```python
from build123d import *

# Parameters (mm, degrees)
F0_R     = 34.9
F0_R_2   = 5.1
F1_DEPTH = 9
F2_R     = 8
F3_DEPTH = 10
F5_DEPTH = 10


# Not quite as in the source:
# - a feature names something its author has since deleted; it is built from what else it names


with BuildPart() as f1:
    # F0 (on Front) → F1 (new body)
    with BuildSketch(Plane.XZ):
        Circle(F0_R)
        Circle(F0_R_2, mode=Mode.SUBTRACT)
    extrude(amount=-F1_DEPTH)

    # F2 (on Front) → F3 (cut)
    with BuildSketch(Plane.XZ):
        with Locations((-16.4184611318, 12.093285839)):
            Circle(F2_R)
        with Locations((-20.4734861558, -5.6729396131)):
            Circle(F2_R)
        with Locations((-9.1115585215, -19.920346226)):
            Circle(F2_R)
        with Locations((9.1115585215, -19.920346226)):
            Circle(F2_R)
        with Locations((20.4734861558, -5.6729396131)):
            Circle(F2_R)
        with BuildLine():
            ThreePointArc((8, 20), (5.6568542495, 25.6568542495), (0, 28))
            Line((0, 28), (0, 12))
            ThreePointArc((0, 12), (5.6568542495, 14.3431457505), (8, 20))
        make_face()
        with BuildLine():
            Line((0, 12), (0, 28))
            ThreePointArc((0, 28), (-8, 20), (0, 12))
        make_face()
        with Locations((16.4184611318, 12.093285839)):
            Circle(F2_R)
    extrude(amount=-F3_DEPTH, mode=Mode.SUBTRACT)

    # F4 (on face) → F5 (cut)
    with BuildSketch(Plane.XZ):
        with BuildLine():
            ThreePointArc((12.2493254993, 32.6797188607), (12.2053527551, 30.4437628813), (13.7203077268, 28.7986658698))
            Line((13.7203077268, 28.7986658698), (15.0106187983, 31.5070043529))
            ThreePointArc((15.0106187983, 31.5070043529), (13.6425787741, 32.1230453786), (12.2493254993, 32.6797188607))
        make_face()
        with BuildLine():
            Line((15.0106187983, 31.5070043529), (13.7203077268, 28.7986658698))
            ThreePointArc((13.7203077268, 28.7986658698), (15.9523075922, 28.6586324994), (17.6609971055, 30.1014813795))
            ThreePointArc((17.6609971055, 30.1014813795), (16.3509172571, 30.8327343071), (15.0106187983, 31.5070043529))
        make_face()
    extrude(amount=-F5_DEPTH, mode=Mode.SUBTRACT)


solid = f1.part
```
The model under review builds one solid part; all positions refer to its coordinate system, in mm. Round coordinates to 2 decimals unless told otherwise and drop trailing zeros. Write each loop counter-clockwise with the first axis right and the second up, starting at its lowest first coordinate (ties: lowest second). Pieces come first, ordered by that corner, then holes.
(1) We need section A-A on x = -23.5. Give the boundary of the cut face in (y, z).
(2) Mouldability with a two-part tool opening along X and no side actions: class faces 1 (the cylindrical face through (-16.34, 4.44, -30.84)), 2 (the cylindrical face through (-15.46, 4.44, -24.79)), 3 (the flat face through (7, 9, 0)) as +X half, -X half, draft (parallel to the pull), parting line (faces both ways), or undercut.
(3) We need section D-D on z = 24.5. Give the boundary of the cut face in (x, y).
(4) We need section C-C on x = -4. Give the boundary of the cut face in (y, z).
(5) We need section B-B on z = 7. Give the boundary of the cut face in (x, y), and give its area (3 significant figures).
(6) Wall thickness on L1, parallel to X at y = 7.25, z = 8; L2, parallel to Z at x = -19.5, y = 3.75; L3, parallel to Z at x = 10, y = 7.75: over which ranges is each line inside the solid? List them lowest first.
(7) Insertion check: pin 1 (1.5 mm diameter, centred on x = -16, z = 4, fed in from -Y); pin 2 (4 mm diameter, centred on y = 3, z = -19, fed in from -X); pin 3 (14.5 mm diameter, centred on x = 16.42, z = 12.09, fed in from +Y); pin 4 (1.5 mm diameter, centred on y = 1.5, z = -21.5, fed in from -X). Each pin has a flat end and moves straight along its axis. Give the tip position at first contact, or say it passes through.
Findings below:
1. outline: (0, -25.8) - (9, -25.8) - (9, -13.08) - (0, -13.08) - close; (0, 1.73) - (9, 1.73) - (9, 8.37) - (0, 8.37) - close; (0, 15.82) - (9, 15.82) - (9, 25.8) - (0, 25.8) - close
2. face 1: parting line
2. face 2: undercut
2. face 3: draft
3. outline: (-24.85, 0) - (-6.61, 0) - (-6.61, 9) - (-24.85, 9) - close; (6.61, 0) - (24.85, 0) - (24.85, 9) - (6.61, 9) - close
4. outline: (0, -34.67) - (9, -34.67) - (9, -26.07) - (0, -26.07) - close; (0, -13.77) - (9, -13.77) - (9, -3.16) - (0, -3.16) - close; (0, 3.16) - (9, 3.16) - (9, 13.07) - (0, 13.07) - close; (0, 26.93) - (9, 26.93) - (9, 34.67) - (0, 34.67) - close
5. outline: (-34.19, 0) - (-22.59, 0) - (-22.59, 9) - (-34.19, 9) - close; (-10.25, 0) - (10.25, 0) - (10.25, 9) - (-10.25, 9) - close; (22.59, 0) - (34.19, 0) - (34.19, 9) - (22.59, 9) - close
5. area: 393 mm2
6. L1: x = -33.97 to -23.29, -9.54 to 9.54, 23.29 to 33.97
6. L2: z = -28.94 to -13.61, 2.27 to 4.71, 19.48 to 28.94
6. L3: z = -33.44 to -27.87, -11.97 to 7.32, 16.87 to 33.44
7. pin 1: stops at y = 0
7. pin 2: stops at x = -30.48
7. pin 3: passes through
7. pin 4: stops at x = -28.06
